Work out the finished part from the listing and answer in its coordinate system (mm). A direction names the side the tool comes from. Round coordinates to 2 decimals unless told otherwise and drop trailing zeros. Order: outer loops, then holes, each group sorted by start corner. A loop starts at its lowest first (then second) coordinate and runs counter-clockwise, first axis right, second up. Notation, with made-up numbers: (30.25, -6) - (61.25, -6) arc R15 cw to (61.25, 1) - close; hole circle Ø2 at (-18.5, 22.5). An arc over 180 degrees is marked (long way). Use CSV: the item, a comma, the result in double quotes.
from build123d import *

# Parameters (mm, degrees)
BOSS_EXTRUDE1_DEPTH = 2.5
SKETCH2_W           = 6.089
SKETCH2_H           = 29.817230859
CUT_EXTRUDE1_DEPTH  = 1


with BuildPart() as part:
    # Sketch1 → Boss-Extrude1 (new body)
    with BuildSketch(Plane(origin=(0, 0, 0), x_dir=(1, 0, 0), z_dir=(0, 1, 0))):
        with BuildLine():
            Line((50, -12.5), (50, -39.143965052))
            ThreePointArc((50, -39.143965052), (63.5, 0), (50, 39.143965052))
            Line((50, 39.143965052), (50, 12.5))
            Line((50, 12.5), (46.5, 12.5))
            Line((46.5, 12.5), (46.5, -12.5))
            Line((46.5, -12.5), (50, -12.5))
        make_face()
    extrude(amount=BOSS_EXTRUDE1_DEPTH)

    # Sketch2 → Cut-Extrude1 (cut)
    with BuildSketch(Plane(origin=(0, 2.5, 0), x_dir=(1, 0, 0), z_dir=(0, 1, 0))):
        with Locations((53.0445, 27.40861543)):
            Rectangle(SKETCH2_W, SKETCH2_H)
        with Locations((53.0445, -27.40861543)):
            Rectangle(SKETCH2_W, SKETCH2_H)
    extrude(amount=-CUT_EXTRUDE1_DEPTH, mode=Mode.SUBTRACT)


solid = part.part
(1) Find section C-C (z = 21). Determine the outline of the cut face in (x, y).
Findings below:
outline,"(50, 0) - (59.93, 0) - (59.93, 2.5) - (56.09, 2.5) - (56.09, 1.5) - (50, 1.5) - close"
(2) Find section D-D (z = -30.5). Determine the outline of the cut face in (x, y).
Findings below:
outline,"(50, 0) - (55.7, 0) - (55.7, 1.5) - (50, 1.5) - close"
(3) Find the intervals of material crossed by L1, parallel to Y at x = 53.5, z = -30; L2, parallel to X at y = 1.35, z = -32; L3, parallel to Z at x = 48.75, y = 1.8, in increasing order. Write a range as from..to.
Findings below:
L1,"y = 0..1.5"
L2,"x = 50..54.85"
L3,"z = -12.5..12.5"
(4) For faces 1 (the flat face through (50, 1, -26)), 2 (the flat face through (53, 1.5, 23)), 3 (the flat face through (53, 1.5, -23)), determine the directions among +Z, -Z, +X, -X, +Y, -Y from which every point of the face is accessible in a straight line to the end or side of a thin tool.
Findings below:
face 1,"-Z, -X, +Y, -Y"
face 2,"+Z, -X, +Y"
face 3,"-Z, -X, +Y"
(5) Find section B-B (x = 54.25). Determine the outline of the cut face in (y, z).
Findings below:
outline,"(0, -33) - (1.5, -33) - (1.5, -12.5) - (2.5, -12.5) - (2.5, 12.5) - (1.5, 12.5) - (1.5, 33) - (0, 33) - close"
(6) Find section A-A (y = 1.95). Determine the outline of the cut face in (x, z).
Findings below:
outline,"(46.5, -12.5) - (56.09, -12.5) - (56.09, -29.77) arc R63.5 ccw to (56.09, 29.77) - (56.09, 12.5) - (46.5, 12.5) - close"
(7) Each of these flat-tipped pins is pushed along its axis until it touches: pin 1 (3 mm diameter, centred on x = 54.5, z = 19.5, fed in from +Y); pin 2 (0.5 mm diameter, centred on y = 2, z = -21, fed in from -X). Where does it stop, or does it pass through?
Findings below:
pin 1,"stops at y = 1.5"
pin 2,"stops at x = 56.09"
